from build123d import *

# Parameters (mm, degrees)
P_IDAT_VYSUNUT_M1_DEPTH  = 1.2
SKICA2_W                 = 35.15
SKICA2_H                 = 28.072940708
P_IDAT_VYSUNUT_M2_DEPTH  = 1.2
LINPOLE1_COUNT           = 2
LINPOLE1_PITCH           = 36.35
SKICA3_W                 = 2.46853356
SKICA3_H                 = 4.337658353
SKICA3_W_2               = 5.363858138
SKICA3_H_2               = 3.395185275
ODEBRAT_VYSUNUT_M1_DEPTH = 47.88381917


with BuildPart() as part:
    # Skica1 → Přidat vysunutím1 (new body)
    with BuildSketch(Plane(origin=(0, 0, 0), x_dir=(0, 0, -1), z_dir=(1, 0, 0))):
        Polygon((0, 0), (0, 20), (19.7, 0), align=None)
    p_idat_vysunut_m1 = extrude(amount=P_IDAT_VYSUNUT_M1_DEPTH)

    # Skica2 → Přidat vysunutím2 (add)
    with BuildSketch(Plane(origin=(0, 9.848875128, -9.998857998), x_dir=(-1, 0, 0), z_dir=(0, 0.7017433693479112, -0.7124298165968641))):
        with Locations((-18.775, 0.212125978)):
            Rectangle(SKICA2_W, SKICA2_H)
    extrude(amount=-P_IDAT_VYSUNUT_M2_DEPTH)

    # LinPole1: Přidat vysunutím1 ×2
    with Locations(*[(i * LINPOLE1_PITCH, 0, 0) for i in range(1, LINPOLE1_COUNT)]):
        add(p_idat_vysunut_m1)

    # Skica3 → Odebrat vysunutím1 (cut, through all)
    with BuildSketch(Plane(origin=(37.55, 0, 0), x_dir=(0, 0, -1), z_dir=(1, 0, 0))):
        with Locations((-1.23426678, 19.003869159)):
            Rectangle(SKICA3_W, SKICA3_H)
        with Locations((19.532023183, -1.697592638)):
            Rectangle(SKICA3_W_2, SKICA3_H_2)
    extrude(amount=-ODEBRAT_VYSUNUT_M1_DEPTH, mode=Mode.SUBTRACT)


solid = part.part
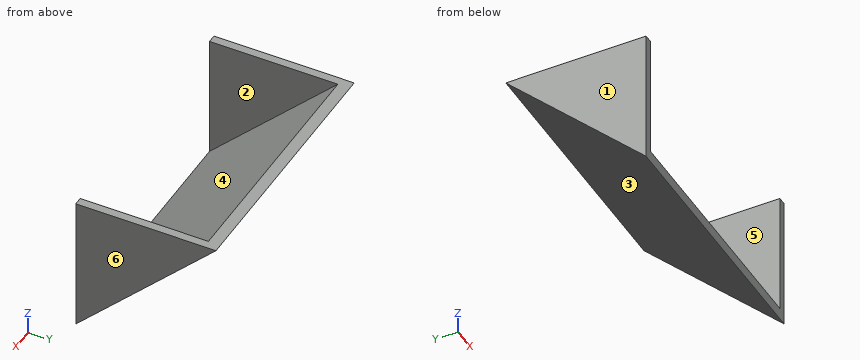
Source: CAD feature listing. Evaluate the final solid. Frame: model axes, mm. Face numbers are marked on the shaded views. A direction names the side the tool comes from. Give positions to 0.01 mm unless a question says otherwise; leave off trailing zeros. Write each loop counter-clockwise with the first axis right and the second up, starting at its lowest first coordinate (ties: lowest second). Pieces come first, ordered by that corner, then holes. Notation, with made-up numbers: M 81,18 L 122,18 A21 cw 122,50 Z; hole C 58,36.5 d1. An arc over 180 degrees is marked long. Return JSON: item names as keys, results as strings. Group by question number.
1) Cut plane A-A, the plane y = 5.5. Output: boundary loops of the cut face in (x, z).
2) Pin query (flat end, axial travel): P1, Ø10, axis at x = 32.5, y = 2.5, coming from the +Z side; P2, Ø2, axis at x = 9.5, y = 13, coming from the -Z side; P3, Ø4, axis at x = 15.5, y = 13, coming from the -Z side (3 decimals); P4, Ø4, axis at x = 30, y = 3.5, coming from the +Z side. Return the tip coordinate at first contact, or that it passes through.
3) Material intervals for line 1 along X through (y, z) = (2, -4); line 2 along Z through (x, y) = (25, 2), sorted ascending. Write a range as [from, to].
4) Pull-direction query (X, two-part tool) for the marked faces 1, 2, 3 and 4; classes: pulls with the +X half, pulls with the -X half, needs draft (parallel to the pull), parting line crosses it, or undercut.
5) Cut plane C-C, the plane x = 3. Output: boundary loops of the cut face in (y, z).
6) Cut plane B-B, the plane z = -13. Output: boundary loops of the cut face in (x, y).
7) Set-up query: the marked faces 5 and 6. Return all of +Z, -Z, +X, -X, +Y, -Y with unobstructed straight access to the full face (end or side cutting, diameter ignored); none if empty.
Recorded:
{
 "1": {"outline": "M 0,-14.28 L 37.55,-14.28 L 37.55,0 L 36.35,0 L 36.35,-12.6 L 1.2,-12.6 L 1.2,0 L 0,0 Z"},
 "2": {"P1": "stops at z = 0", "P2": "stops at z = -7.88", "P3": "stops at z = -8.865", "P4": "stops at z = -12.6"},
 "3": {"line 1": "x = [0, 1.2], [36.35, 37.55]", "line 2": "z = [-17.73, -16.05]"},
 "4": {"face 1": "pulls with the -X half", "face 2": "undercut", "face 3": "needs draft", "face 4": "undercut"},
 "5": {"outline": "M 0,-19.7 L 20,0 L 18.29,0 L 0,-18.02 Z"},
 "6": {"outline": "M 0,0 L 1.2,0 L 1.2,5.09 L 36.35,5.09 L 36.35,0 L 37.55,0 L 37.55,6.8 L 0,6.8 Z"},
 "7": {"face 5": "+Z, -Y", "face 6": "+Z, -Z, +X, +Y, -Y"}
}
